For this review, use the dimensioned drawing (mm, ordinates from the lowest corner) and the shaded views. A direction names the side the tool comes from. Coordinates: 2 decimals unless noted, no trailing zeros. Loops run counter-clockwise (first coordinate to the right, second up) from the corner with the lowest first, then second, coordinate; pieces in that order, holes last. Notation, with made-up numbers: M -7.5,84.5 L 34.5,84.5 A34 ccw 34.5,115.5 Z; hole C 38,-14 d7. An arc over 180 degrees is marked long. One line per item, written item: value.
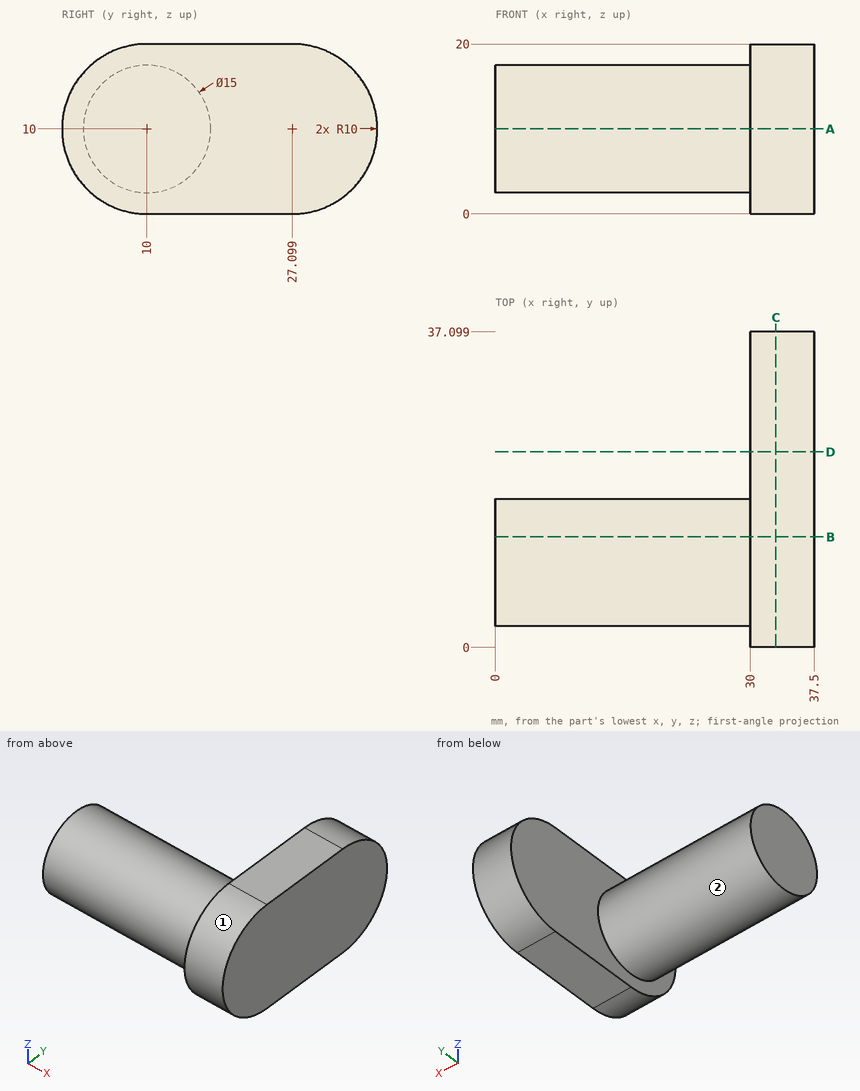
(1) We need section C-C on x = 33. State the section outline as (y, z) points.
Reply:
outline: M 10,0 L 27.1,0 A10 ccw 27.1,20 L 10,20 A10 ccw Z
(2) Insertion check: pin 1 (1.5 mm diameter, centred on x = 9, z = 13.5, fed in from +Y); pin 2 (8 mm diameter, centred on y = 31, z = 9.5, fed in from -X); pin 3 (1 mm diameter, centred on x = 26, y = 8, fed in from -Z); pin 4 (5 mm diameter, centred on x = 31.5, y = 20.5, fed in from -Z). Each pin has a flat end and moves straight along its axis. Give the tip position at first contact, or say it passes through.
Reply:
pin 1: stops at y = 16.98
pin 2: stops at x = 30
pin 3: stops at z = 2.65
pin 4: stops at z = 0
(3) Tool access review of the marked faces 1 and 2: name each direction out of +Z, -Z, +X, -X, +Y, -Y from which nothing blocks a thin tool from reaching the whole face with its end or side.
Reply:
face 1: +X, -X, -Y
face 2: -X
(4) We need section A-A on z = 10. State the section outline as (x, y) points, then the cut area to 3 significant figures.
Reply:
outline: M 0,2.5 L 30,2.5 L 30,0 L 37.5,0 L 37.5,37.1 L 30,37.1 L 30,17.5 L 0,17.5 Z
area: 728 mm2
(5) To check wall thickness, follow line 1 along X through (y, z) = (22, 9.25); line 2 along Z through (x, y) = (13.5, 10); line 3 along Y through (x, z) = (25.5, 7.25). State the ranges of each line that lie inside material, in increasing order. Write a range as [from, to].
Reply:
line 1: x = [30, 37.5]
line 2: z = [2.5, 17.5]
line 3: y = [3.02, 16.98]
(6) We need section D-D on y = 23. State the section outline as (x, z) points, then the cut area to 3 significant figures.
Reply:
outline: M 30,0 L 37.5,0 L 37.5,20 L 30,20 Z
area: 150 mm2
(7) We need section B-B on y = 13. State the section outline as (x, z) points.
Reply:
outline: M 0,3.13 L 30,3.13 L 30,0 L 37.5,0 L 37.5,20 L 30,20 L 30,16.87 L 0,16.87 Z
